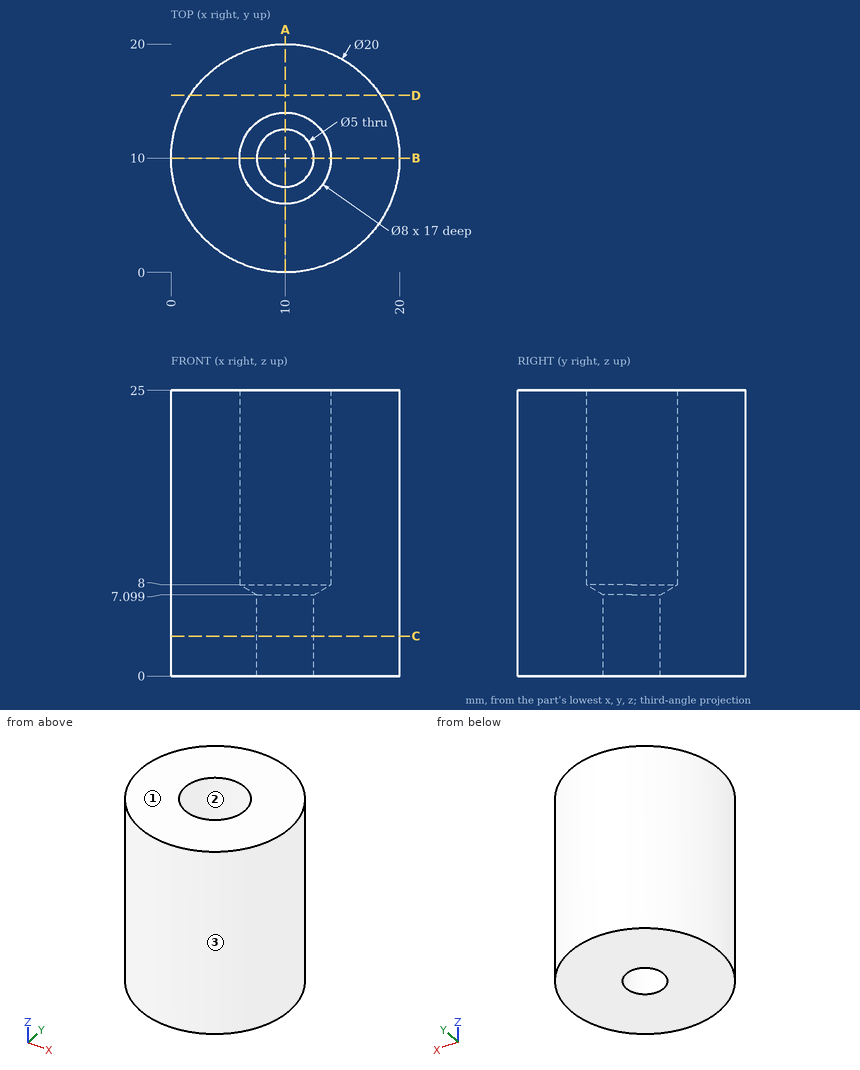
For this review, use the dimensioned drawing (mm, ordinates from the lowest corner) and the shaded views. Coordinates: 2 decimals unless noted, no trailing zeros. Write each loop counter-clockwise with the first axis right and the second up, starting at its lowest first coordinate (ties: lowest second). Pieces come first, ordered by that corner, then holes. Notation, with made-up numbers: (-10, 4) -> (38, 4) arc R24 cw to (38, 18) -> close; hole circle Ø10 at (45, 58). An arc over 180 degrees is marked (long way). Put each result on its own line as item: value.
Q1. Wall thickness on L1, parallel to Y at x = 10, z = 2.25; L2, parallel to Y at x = 10, z = 19; L3, parallel to X at y = 9.75, z = 7.5 (1 decimal): over which ranges is each line inside the solid? List them lowest first.
From the geometry:
L1: y = 0 to 7.5, 12.5 to 20
L2: y = 0 to 6, 14 to 20
L3: x = 0 to 6.8, 13.2 to 20
Q2. Clearance check with flat-ended pins moving along their axes: pin 1 Ø2 at (x, y) = (7.5, 12.5) entering from +Z; pin 2 Ø1 at (y, z) = (13, 16) entering from +X; pin 3 Ø1.5 at (y, z) = (3.5, 16) entering from -X; pin 4 Ø4 at (y, z) = (16, 12) entering from -X (1 decimal). State where each tip first meets the part, or that it passes through.
From the geometry:
pin 1: stops at z = 25
pin 2: stops at x = 19.68
pin 3: stops at x = 1.82
pin 4: stops at x = 0.8
Q3. Take a section at A-A, the plane x = 10. State the section outline as (y, z) points.
From the geometry:
outline: (0, 0) -> (7.5, 0) -> (7.5, 7.1) -> (6, 8) -> (6, 25) -> (0, 25) -> close; (12.5, 0) -> (20, 0) -> (20, 25) -> (14, 25) -> (14, 8) -> (12.5, 7.1) -> close
Q4. Take a section at D-D, the plane y = 15.5. State the section outline as (x, z) points.
From the geometry:
outline: (1.65, 0) -> (18.35, 0) -> (18.35, 25) -> (1.65, 25) -> close
Q5. Take a section at C-C, the plane z = 3.5. State the section outline as (x, y) points.
From the geometry:
outline: circle Ø20 at (10, 10); hole circle Ø5 at (10, 10)
Q6. The part is to be moulded in two halves that separate along Y. For the marked faces 1, 2 and 3, say which applies: +Y half, -Y half, draft (parallel to the pull), parting line (faces both ways), or undercut.
From the geometry:
face 1: draft
face 2: undercut
face 3: parting line
